CAD build for the part. Positions are in the model's coordinates, mm. Round coordinates to 2 decimals unless told otherwise and drop trailing zeros. Write each loop counter-clockwise with the first axis right and the second up, starting at its lowest first coordinate (ties: lowest second). Pieces come first, ordered by that corner, then holes. Notation, with made-up numbers: (29.5, 13.5) -> (64.5, 13.5) arc R14 cw to (64.5, 22.5) -> close; hole circle Ø5 at (-25, 36). An arc over 180 degrees is marked (long way). Answer in a Markdown table with one row per item. Add a question column.
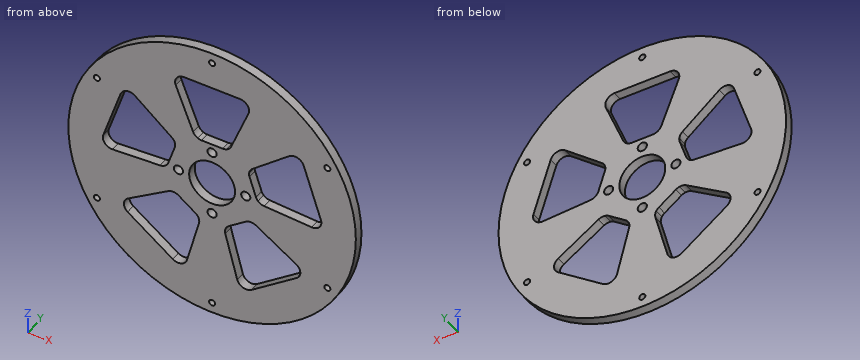
```python
from build123d import *

# Parameters (mm, degrees)
F0_R     = 47
F0_R_2   = 7.5
F1_DEPTH = 3
F3_D     = 2
F5_D     = 3


with BuildPart() as f1:
    # F0 (on Front) → F1 (new body)
    with BuildSketch(Plane.XZ):
        Circle(F0_R)
        with BuildLine():
            ThreePointArc((13.499536, 34.44942), (30.565363, 20.850865), (37, 0))
            ThreePointArc((37, 0), (1.097165, -36.983729), (-36.934931, -2.193365))
            ThreePointArc((-36.934931, -2.193365), (-35.189091, 11.433629), (-28.591759, 23.484278))
            ThreePointArc((-28.591759, 23.484278), (-21.748054, 29.933629), (-13.499536, 34.44942))
            ThreePointArc((-13.499536, 34.44942), (-6.869187, 36.356764), (0, 37))
            ThreePointArc((0, 37), (6.869187, 36.356764), (13.499536, 34.44942))
        make_face(mode=Mode.SUBTRACT)
        with BuildLine():
            ThreePointArc((-36.934931, -2.193365), (1.097165, -36.983729), (37, 0))
            ThreePointArc((37, 0), (30.565363, 20.850865), (13.499536, 34.44942))
            ThreePointArc((13.499536, 34.44942), (6.869187, 36.356764), (0, 37))
            ThreePointArc((0, 37), (-6.869187, 36.356764), (-13.499536, 34.44942))
            ThreePointArc((-13.499536, 34.44942), (-21.748054, 29.933629), (-28.591759, 23.484278))
            ThreePointArc((-28.591759, 23.484278), (-35.189091, 11.433629), (-36.934931, -2.193365))
        make_face()
        with BuildLine():
            ThreePointArc((4.693528, 14.246782), (5.085095, 14.111761), (5.472785, 13.965981))
            ThreePointArc((5.472785, 13.965981), (8.816779, 12.135255), (11.591254, 9.520653))
            ThreePointArc((11.591254, 9.520653), (11.849702, 9.196987), (12.099115, 8.866309))
            ThreePointArc((12.099115, 8.866309), (12.447774, 9.946358), (13.172702, 10.8196))
            Line((13.172702, 10.8196), (25.193427, 20.693005))
            ThreePointArc((25.193427, 20.693005), (27.939595, 21.254159), (29.950727, 19.301805))
            Line((29.950727, 19.301805), (35.575964, 1.989107))
            ThreePointArc((35.575964, 1.989107), (35.096489, -0.772494), (32.544954, -1.932668))
            Line((32.544954, -1.932668), (17.016541, -1.01052))
            ThreePointArc((17.016541, -1.01052), (15.916783, -0.730155), (14.999875, -0.061313))
            ThreePointArc((14.999875, -0.061313), (14.265848, -4.635255), (12.171193, -8.767102))
            ThreePointArc((12.171193, -8.767102), (13.306123, -8.764943), (14.360639, -9.184544))
            Line((14.360639, -9.184544), (27.465415, -17.565883))
            ThreePointArc((27.465415, -17.565883), (28.847716, -20.004238), (27.612391, -22.520248))
            Line((27.612391, -22.520248), (12.885331, -33.220084))
            ThreePointArc((12.885331, -33.220084), (10.110726, -33.617458), (8.218867, -31.549318))
            Line((8.218867, -31.549318), (4.297339, -16.49596))
            ThreePointArc((4.297339, -16.49596), (4.224138, -15.363391), (4.576904, -14.284675))
            ThreePointArc((4.576904, -14.284675), (0, -15), (-4.576904, -14.284675))
            ThreePointArc((-4.576904, -14.284675), (-4.224138, -15.363391), (-4.297339, -16.49596))
            Line((-4.297339, -16.49596), (-8.218867, -31.549318))
            ThreePointArc((-8.218867, -31.549318), (-10.110726, -33.617458), (-12.885331, -33.220084))
            Line((-12.885331, -33.220084), (-27.612391, -22.520248))
            ThreePointArc((-27.612391, -22.520248), (-28.847716, -20.004238), (-27.465415, -17.565883))
            Line((-27.465415, -17.565883), (-14.360639, -9.184544))
            ThreePointArc((-14.360639, -9.184544), (-13.306123, -8.764943), (-12.171193, -8.767102))
            ThreePointArc((-12.171193, -8.767102), (-14.132429, -5.02737), (-14.973621, -0.889202))
            ThreePointArc((-14.973621, -0.889202), (-14.992463, -0.475439), (-14.999875, -0.061313))
            ThreePointArc((-14.999875, -0.061313), (-15.916783, -0.730155), (-17.016541, -1.01052))
            Line((-17.016541, -1.01052), (-32.544954, -1.932668))
            ThreePointArc((-32.544954, -1.932668), (-35.096489, -0.772494), (-35.575964, 1.989107))
            Line((-35.575964, 1.989107), (-29.950727, 19.301805))
            ThreePointArc((-29.950727, 19.301805), (-27.939595, 21.254159), (-25.193427, 20.693005))
            Line((-25.193427, 20.693005), (-13.172702, 10.8196))
            ThreePointArc((-13.172702, 10.8196), (-12.447774, 9.946358), (-12.099115, 8.866309))
            ThreePointArc((-12.099115, 8.866309), (-9.148474, 11.887196), (-5.472785, 13.965981))
            ThreePointArc((-5.472785, 13.965981), (-5.085095, 14.111761), (-4.693528, 14.246782))
            ThreePointArc((-4.693528, 14.246782), (-5.612975, 14.91213), (-6.219462, 15.871424))
            Line((-6.219462, 15.871424), (-11.89502, 30.354863))
            ThreePointArc((-11.89502, 30.354863), (-11.580097, 33.140031), (-9.101824, 34.44942))
            Line((-9.101824, 34.44942), (9.101824, 34.44942))
            ThreePointArc((9.101824, 34.44942), (11.580097, 33.140031), (11.89502, 30.354863))
            Line((11.89502, 30.354863), (6.219462, 15.871424))
            ThreePointArc((6.219462, 15.871424), (5.612975, 14.91213), (4.693528, 14.246782))
        make_face(mode=Mode.SUBTRACT)
        with BuildLine():
            ThreePointArc((11.591254, 9.520653), (8.816779, 12.135255), (5.472785, 13.965981))
            ThreePointArc((5.472785, 13.965981), (5.085095, 14.111761), (4.693528, 14.246782))
            ThreePointArc((4.693528, 14.246782), (4.075266, 14.037022), (3.426266, 13.965981))
            Line((3.426266, 13.965981), (-3.426266, 13.965981))
            ThreePointArc((-3.426266, 13.965981), (-4.075266, 14.037022), (-4.693528, 14.246782))
            ThreePointArc((-4.693528, 14.246782), (-5.085095, 14.111761), (-5.472785, 13.965981))
            ThreePointArc((-5.472785, 13.965981), (-9.148474, 11.887196), (-12.099115, 8.866309))
            ThreePointArc((-12.099115, 8.866309), (-12.090675, 8.213486), (-12.223663, 7.574298))
            Line((-12.223663, 7.574298), (-14.341212, 1.057153))
            ThreePointArc((-14.341212, 1.057153), (-14.609328, 0.46187), (-14.999875, -0.061313))
            ThreePointArc((-14.999875, -0.061313), (-14.992463, -0.475439), (-14.973621, -0.889202))
            ThreePointArc((-14.973621, -0.889202), (-14.132429, -5.02737), (-12.171193, -8.767102))
            ThreePointArc((-12.171193, -8.767102), (-11.547714, -8.960809), (-10.980905, -9.284808))
            Line((-10.980905, -9.284808), (-5.437091, -13.312624))
            ThreePointArc((-5.437091, -13.312624), (-4.953796, -13.751571), (-4.576904, -14.284675))
            ThreePointArc((-4.576904, -14.284675), (0, -15), (4.576904, -14.284675))
            ThreePointArc((4.576904, -14.284675), (4.953796, -13.751571), (5.437091, -13.312624))
            Line((5.437091, -13.312624), (10.980905, -9.284808))
            ThreePointArc((10.980905, -9.284808), (11.547714, -8.960809), (12.171193, -8.767102))
            ThreePointArc((12.171193, -8.767102), (14.265848, -4.635255), (14.999875, -0.061313))
            ThreePointArc((14.999875, -0.061313), (14.609328, 0.46187), (14.341212, 1.057153))
            Line((14.341212, 1.057153), (12.223663, 7.574298))
            ThreePointArc((12.223663, 7.574298), (12.090675, 8.213486), (12.099115, 8.866309))
            ThreePointArc((12.099115, 8.866309), (11.849702, 9.196987), (11.591254, 9.520653))
        make_face()
        Circle(F0_R_2, mode=Mode.SUBTRACT)
    extrude(amount=F1_DEPTH)

    # F3 (through all)
    with Locations(Plane.XZ.offset(3)):
        with Locations((37.672105, 21.75), (37.672105, -21.75), (0, -43.5), (-37.672105, -21.75), (-37.672105, 21.75), (0, 43.5)):
            Hole(F3_D / 2)

    # F5 (through all)
    with Locations(Plane(origin=(0, 0, 0), x_dir=(1, 0, 0), z_dir=(0, 1, 0))):
        with Locations((0, 11), (11, 0), (0, -11), (-11, 0)):
            Hole(F5_D / 2)


solid = f1.part
```
Item 1: Saw through at C-C on z = 36.5. Give the cut face in (x, y).
Item 2: Pin check, flat tips, straight feed: pin 1 (3 mm diameter, centred on x = 32, z = 18.5, fed in from +Y); pin 2 (1.5 mm diameter, centred on x = -4.5, y = -2, fed in from -Z); pin 3 (1.5 mm diameter, centred on y = -2.5, z = 25, fed in from +X); pin 4 (1.5 mm diameter, centred on x = 0.5, y = -1, fed in from +Z). Stop position of each tip, or through.
Item 3: Drill centre lines: probe 1 along Z at (x, y) = (3.5, -0.5); probe 2 along Z at (x, y) = (21, -1.2); probe 3 along X at (y, z) = (-0.25, -26.5). Where is each one in solid material? Low to high.
Item 4: Saw through at B-B on y = -2.2. Count the separate pieces of the cut face and the enclosed holes in it, then the cut area to 3 significant figures.
Item 5: Saw through at A-A on z = -4. Give the cut face in (x, y), then the cut area to 3 significant figures.
Recorded:
| question | item | result |
|---|---|---|
| 1 | outline | (-29.61, -3) -> (29.61, -3) -> (29.61, 0) -> (-29.61, 0) -> close |
| 2 | pin 1 | y = 0 |
| 2 | pin 2 | z = -46.85 |
| 2 | pin 3 | x = 40.26 |
| 2 | pin 4 | z = 47 |
| 3 | probe 1 | -46.87 to -6.63, 6.63 to 13.97, 34.45 to 46.87 |
| 3 | probe 2 | -42.05 to -27.32, -13.43 to -1.25, 17.25 to 42.05 |
| 3 | probe 3 | -38.82 to -22.13, -6.9 to 6.9, 22.13 to 38.82 |
| 4 | separate pieces | 1 |
| 4 | enclosed holes | 16 |
| 4 | area | 4,820 mm2 |
| 5 | outline | (-46.83, -3) -> (-6.34, -3) -> (-6.34, 0) -> (-46.83, 0) -> close; (6.34, -3) -> (46.83, -3) -> (46.83, 0) -> (6.34, 0) -> close |
| 5 | area | 243 mm2 |
